```python
from build123d import *

# Parameters (mm, degrees)
F0_W        = 58.42
F0_H        = 101.6
F1_DEPTH    = 3.81
F2_T1_DEPTH = 126.1934442484
F2_T3_DEPTH = 83.0134442484
F4_T        = -2.54
F3_R        = 2.0082426315
F5_DEPTH    = 25.4


# Not quite as in the source:
# - a fillet or chamfer that OpenCascade refuses, or shapes differently, is made with other operations: its cross-section is extruded or revolved along the edge and cut away or added


with BuildPart() as f1:
    # F0 (on Front) → F1 (new body)
    with BuildSketch(Plane.XZ):
        Rectangle(F0_W, F0_H)
    extrude(amount=F1_DEPTH)

    # F2: fillet of radius 5.08 on 4 edges, made by hand

    # F2_s2 → F2_t1 (cut)
    with BuildSketch(Plane.XY.offset(-63.0967221242)):
        with BuildLine():
            ThreePointArc((-29.21, 0), (-27.4021631237, -2.7460926284), (-24.2913111503, -3.81))
            Line((-24.2913111503, -3.81), (-24.2913111503, -3.9116))
            Line((-24.2913111503, -3.9116), (-29.21, -3.9116))
            Line((-29.21, -3.9116), (-29.3116, -3.81))
            ThreePointArc((-29.3116, -3.81), (-29.3116, -1.905), (-29.308373777, -0.0254))
            Line((-29.308373777, -0.0254), (-29.21, 0))
        make_face()
        with BuildLine():
            ThreePointArc((29.21, 0), (27.4021631237, -2.7460926284), (24.2913111503, -3.81))
            Line((24.2913111503, -3.81), (24.2913111503, -3.9116))
            Line((24.2913111503, -3.9116), (29.21, -3.9116))
            Line((29.21, -3.9116), (29.3116, -3.81))
            ThreePointArc((29.3116, -3.81), (29.3116, -1.905), (29.308373777, -0.0254))
            Line((29.308373777, -0.0254), (29.21, 0))
        make_face()
    extrude(amount=F2_T1_DEPTH, mode=Mode.SUBTRACT)

    # F2_s4 → F2_t3 (cut)
    with BuildSketch(Plane.YZ.offset(-41.5067221242)):
        with BuildLine():
            ThreePointArc((0, 50.8), (-2.7460926284, 48.9921631237), (-3.81, 45.8813111503))
            Line((-3.81, 45.8813111503), (-3.9116, 45.8813111503))
            Line((-3.9116, 45.8813111503), (-3.9116, 50.8))
            Line((-3.9116, 50.8), (-3.81, 50.9016))
            ThreePointArc((-3.81, 50.9016), (-1.905, 50.9016), (-0.0254, 50.898373777))
            Line((-0.0254, 50.898373777), (0, 50.8))
        make_face()
        with BuildLine():
            ThreePointArc((0, -50.8), (-2.7460926284, -48.9921631237), (-3.81, -45.8813111503))
            Line((-3.81, -45.8813111503), (-3.9116, -45.8813111503))
            Line((-3.9116, -45.8813111503), (-3.9116, -50.8))
            Line((-3.9116, -50.8), (-3.81, -50.9016))
            ThreePointArc((-3.81, -50.9016), (-1.905, -50.9016), (-0.0254, -50.898373777))
            Line((-0.0254, -50.898373777), (0, -50.8))
        make_face()
    extrude(amount=F2_T3_DEPTH, mode=Mode.SUBTRACT)

    # F4
    f4_openings = [f1.faces().sort_by_distance(p)[0] for p in [
        (0, 0, 0),
    ]]
    offset(amount=F4_T, openings=f4_openings)

    # F3 (on face) → F5 (cut)
    with BuildSketch(Plane(origin=(0, 0, 0), x_dir=(-1, 0, 0), z_dir=(0, 1, 0))):
        with BuildLine():
            Line((10.0412131573, 34.8095389452), (-10.0412131573, 34.8095389452))
            ThreePointArc((-10.0412131573, 34.8095389452), (-17.399, 19.413012104), (-10.0412131573, 4.0164852629))
            Line((-10.0412131573, 4.0164852629), (10.0412131573, 4.0164852629))
            ThreePointArc((10.0412131573, 4.0164852629), (17.399, 19.413012104), (10.0412131573, 34.8095389452))
        make_face()
        with BuildLine():
            Line((10.0412131573, -4.0164852629), (-10.0412131573, -4.0164852629))
            ThreePointArc((-10.0412131573, -4.0164852629), (-17.399, -19.413012104), (-10.0412131573, -34.8095389452))
            Line((-10.0412131573, -34.8095389452), (10.0412131573, -34.8095389452))
            ThreePointArc((10.0412131573, -34.8095389452), (17.399, -19.413012104), (10.0412131573, -4.0164852629))
        make_face()
        Circle(F3_R)
    extrude(amount=-F5_DEPTH, mode=Mode.SUBTRACT)


solid = f1.part
```
Model file for the job. Use its own axes, mm. A direction names the side the tool comes from. Coordinates: 2 decimals unless noted, no trailing zeros. Write each loop counter-clockwise with the first axis right and the second up, starting at its lowest first coordinate (ties: lowest second). Pieces come first, ordered by that corner, then holes. Notation, with made-up numbers: (54.25, 81) - (112.25, 81) arc R19 cw to (112.25, 91) - close; hole circle Ø7 at (49.5, 62.25). An arc over 180 degrees is marked (long way). One line per item, written item: value. Start each with the question number.
1. Slice it at D-D (y = -1.95). Write the cut outline in (x, z).
2. Tool access for faces 1 (the cylindrical face through (-17.397, -2.522, -19.66)), 2 (the cylindrical face through (25.58, -0.92, -0.67)), 3 (the flat face through (-28, 0, 0)): list every direction of +Z, -Z, +X, -X, +Y, -Y with a clear straight run to the whole face (end or side of a thin tool).
3. Slice it at A-A (x = 0). Write the cut outline in (y, z).
4. Flat gauge pins, fed straight in: pin 1 (0.8 mm diameter, centred on x = 0.5, y = -2.5, fed in from +Z); pin 2 (24.5 mm diameter, centred on x = -2, z = 11.5, fed in from +Y); pin 3 (1.5 mm diameter, centred on y = -2.5, z = -1, fed in from +X). Where does each tip first touch, or does it go through?
5. Probe line 1 (Z direction, x = 0, y = -2.35); line 2 (Z direction, x = 0, y = -2.65); line 3 (Z direction, x = -6.5, y = -2.2). List the from-to ranges inside material, lowest first. Write a range as from..to.
6. Slice it at C-C (z = 39). Write the cut outline in (x, y), plus the area to 3 significant figures.
7. Slice it at B-B (z = 0). Write the cut outline in (x, y), plus the area to 3 significant figures.
8. Mould opens along X. For faces 4 (the cylindrical face through (17.397, -2.522, -19.166)), 5 (the cylindrical face through (-27.439, -2.717, -0.711)), 6 (the flat face through (5, -3.81, 1)) say: released by +X, released by -X, zero draft, split by the parting line, or undercut.
Answers below:
1. outline: (-28.22, -49.81) - (28.22, -49.81) - (28.22, 49.81) - (-28.22, 49.81) - close; hole (-10.04, -34.81) - (10.04, -34.81) arc R19.79 ccw to (10.04, -4.02) - (-10.04, -4.02) arc R19.79 ccw to start; hole (-10.04, 4.02) - (10.04, 4.02) arc R19.79 ccw to (10.04, 34.81) - (-10.04, 34.81) arc R19.79 ccw to start; hole circle Ø4.02 at (0, 0)
2. face 1: +Y, -Y
2. face 2: +Y
2. face 3: +Z, -Z, +X, -X, +Y
3. outline: (-3.81, -45.88) arc R5.08 ccw to (0, -50.8) - (0, -48.08) arc R2.54 cw to (-1.27, -45.88) - (-1.27, -34.81) - (-3.81, -34.81) - close; (-3.81, -4.02) - (-1.27, -4.02) - (-1.27, -2.01) - (-3.81, -2.01) - close; (-3.81, 2.01) - (-1.27, 2.01) - (-1.27, 4.02) - (-3.81, 4.02) - close; (-3.81, 34.81) - (-1.27, 34.81) - (-1.27, 45.88) arc R2.54 cw to (0, 48.08) - (0, 50.8) arc R5.08 ccw to (-3.81, 45.88) - close
4. pin 1: stops at z = 49.68
4. pin 2: stops at y = -1.27
4. pin 3: stops at x = 28.38
5. line 1: z = -49.45..-34.81, -4.02..-2.01, 2.01..4.02, 34.81..49.45
5. line 2: z = -49.11..-34.81, -4.02..-2.01, 2.01..4.02, 34.81..49.11
5. line 3: z = -49.59..-34.81, -4.02..4.02, 34.81..49.59
6. outline: (-29.21, 0) arc R5.08 ccw to (-24.29, -3.81) - (24.29, -3.81) arc R5.08 ccw to (29.21, 0) - (26.49, 0) arc R2.54 cw to (24.29, -1.27) - (-24.29, -1.27) arc R2.54 cw to (-26.49, 0) - close
6. area: 147 mm^2
7. outline: (-29.21, 0) arc R5.08 ccw to (-24.29, -3.81) - (-2.01, -3.81) - (-2.01, -1.27) - (-24.29, -1.27) arc R2.54 cw to (-26.49, 0) - close; (2.01, -3.81) - (24.29, -3.81) arc R5.08 ccw to (29.21, 0) - (26.49, 0) arc R2.54 cw to (24.29, -1.27) - (2.01, -1.27) - close
7. area: 137 mm^2
8. face 4: undercut
8. face 5: released by -X
8. face 6: zero draft
